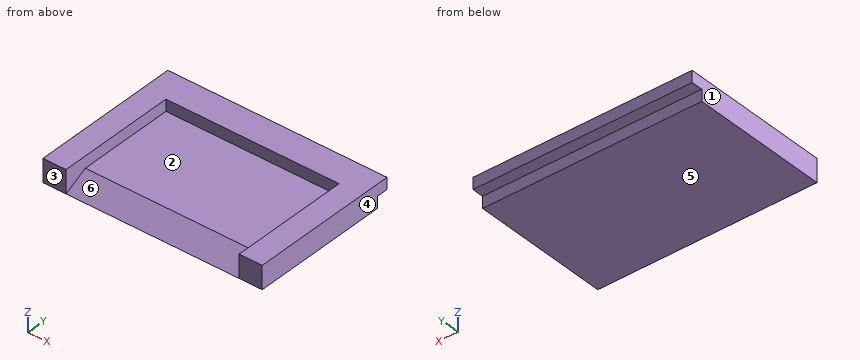
from build123d import *

# Parameters (mm, degrees)
SKETCH1_W           = 95
SKETCH1_H           = 60
BOSS_EXTRUDE1_DEPTH = 10
CUT_EXTRUDE1_DEPTH  = 5
CUT_EXTRUDE2_DEPTH  = 75
SKETCH7_W           = 95
SKETCH7_H           = 5
BOSS_EXTRUDE3_DEPTH = 5


with BuildPart() as part:
    # Sketch1 → Boss-Extrude1 (new body)
    with BuildSketch(Plane.XY):
        with Locations((47.5, 30)):
            Rectangle(SKETCH1_W, SKETCH1_H)
    extrude(amount=BOSS_EXTRUDE1_DEPTH)

    # Sketch2 → Cut-Extrude1 (cut)
    with BuildSketch(Plane.XY.offset(10)):
        Polygon((10, 50), (10, 52), (85, 52), (85, 50), (85, 10), (10, 10), align=None)
    extrude(amount=-CUT_EXTRUDE1_DEPTH, mode=Mode.SUBTRACT)

    # Sketch4 → Cut-Extrude2 (cut)
    with BuildSketch(Plane(origin=(10, 0, 0), x_dir=(0, 0, -1), z_dir=(1, 0, 0))):
        Polygon((0, 0), (-5, 10), (-10, 10), (-10, 0), align=None)
    extrude(amount=CUT_EXTRUDE2_DEPTH, mode=Mode.SUBTRACT)

    # Sketch7 → Boss-Extrude3 (add)
    with BuildSketch(Plane(origin=(0, 60, 0), x_dir=(1, 0, 0), z_dir=(0, 1, 0))):
        with Locations((47.5, -7.5)):
            Rectangle(SKETCH7_W, SKETCH7_H)
    extrude(amount=BOSS_EXTRUDE3_DEPTH)


solid = part.part
Verification items for the finished model (mm, model axes). Face numbers are marked on the shaded views. A direction names the side the tool comes from. Give positions to 0.01 mm unless a question says otherwise; leave off trailing zeros. Loops run counter-clockwise (first coordinate to the right, second up) from the corner with the lowest first, then second, coordinate; pieces in that order, holes last. Notation, with made-up numbers: (8.5, 62.5) - (36.5, 62.5) arc R29 ccw to (36.5, 95.5) - close; hole circle Ø2 at (-11, -3). An arc over 180 degrees is marked (long way). Write item = value, one per line. Start each with the question number.
Q1. Cross-section at A-A, the plane z = 2.25. Enter the section's corners in (x, y), and give its area (3 significant figures).
Q2. Cross-section at B-B, the plane y = 11. Enter the section's corners in (x, z).
Q3. Depth check by flat-ended pin: P1, Ø5.5, axis at x = 58.5, y = 63.5, coming from the -Z side; P2, Ø4, axis at x = 25, z = 2.5, coming from the +Y side; P3, Ø8, axis at x = 52, y = 47, coming from the +Z side. Enter the tip coordinate at first touch or a pass-through.
Q4. Mould release check, pull along X, two halves, no side actions. Record for the marked faces 1, 2, 3 and 4: released by +X, released by -X, zero draft, split by the parting line, or undercut.
Q5. Tool access check on the marked faces 5 and 6. Record the directions out of +Z, -Z, +X, -X, +Y, -Y that give a thin tool (end or side, any length) a straight path to the whole face; none if there is none.
Q6. Thickness scan on line 1 (X direction, y = 23.5, z = 6); line 2 (Y direction, x = 22, z = 7); line 3 (Y direction, x = 60, z = 2.5). Record the ranges inside material, lowest first.
Answer key:
q1.outline = (0, 0) - (10, 0) - (10, 4.5) - (85, 4.5) - (85, 0) - (95, 0) - (95, 60) - (0, 60) - close
q1.area = 5,360 mm^2
q2.outline = (0, 0) - (95, 0) - (95, 10) - (85, 10) - (85, 5) - (10, 5) - (10, 10) - (0, 10) - close
q3.P1 = 5
q3.P2 = 60
q3.P3 = 5
q4.face_1 = released by -X
q4.face_2 = undercut
q4.face_3 = zero draft
q4.face_4 = released by +X
q5.face_5 = -Z, +X, -X, +Y, -Y
q5.face_6 = +Z, -Y
q6.line_1 = 0 to 10, 85 to 95
q6.line_2 = 52 to 65
q6.line_3 = 5 to 60
